Build history of the part. All positions in model axes, mm. A direction names the side the tool comes from. Coordinates: 2 decimals unless noted, no trailing zeros. Write item = value, one per line. Start each with the question number.
Q1. 3-axis set-ups, long thin cutter, end or side, ignore diameter. For faces 4 (the face through (-9.563, -21.028, 0.601)), 5 (the face through (9.854, -21.197, 6.399)), 6 (the face through (13.43, 19.13, 6.4)), 7 (the face through (-13.43, 18.8, 0.6)), 8 (the face through (9.78, -21.81, 3.48)): which of +Z, -Z, +X, -X, +Y, -Y reach the whole face in a straight line?
Q2. Band-saw the part on A-A on z = 6. State how many separate pieces and enclosed holes the cut face has, plus the area to 3 significant figures.
Q3. Drill centre lines: probe 1 along Y at (x, z) = (-0.5, 5.25); probe 2 along Y at (x, z) = (-10, 2.25); probe 3 along Y at (x, z) = (3, 5.25). Where is each one in solid material? Low to high.
Q4. Pin check, flat tips, straight feed: P1, Ø0.7, axis at x = 14.5, z = 3.5, coming from the +Y side; P2, Ø1.1, axis at y = -6.5, z = 3.5, coming from the -X side; P3, Ø1.1, axis at y = 15, z = 3, coming from the -X side; P4, Ø13, axis at x = -26.85, y = -15.5, coming from the +Z side. Stop position of each tip, or through.
Q5. Pull direction X, two halves, no side cores. Call faces 1 (the face through (9.854, -21.197, 0.601)), 2 (the face through (-13.43, 18.8, 6.4)), 3 (the face through (14, 19, 3)): released by +X, released by -X, zero draft, split by the parting line, or undercut.
```python
from build123d import *

# Parameters (mm, degrees)
F0_W     = 1.3256371551
F0_H     = 1.3256371551
F1_DEPTH = 7
F2_R     = 2


with BuildPart() as f1:
    # F0 (on Top) → F1 (new body)
    with BuildSketch(Plane.XY):
        with BuildLine():
            Line((0, 20.1), (0, 17))
            ThreePointArc((0, 17), (9.8994949366, 21.1005050634), (14, 31))
            ThreePointArc((14, 31), (9.8994949366, 40.8994949366), (0, 45))
            Line((0, 45), (0, 41.9))
            ThreePointArc((0, 41.9), (7.7074639149, 38.7074639149), (10.9, 31))
            ThreePointArc((10.9, 31), (7.7074639149, 23.2925360851), (0, 20.1))
        make_face()
        with BuildLine():
            ThreePointArc((-14, 31), (-9.8994949366, 21.1005050634), (0, 17))
            Line((0, 17), (0, 20.1))
            ThreePointArc((0, 20.1), (-10.9, 31), (0, 41.9))
            Line((0, 41.9), (0, 45))
            ThreePointArc((0, 45), (-9.8994949366, 40.8994949366), (-14, 31))
        make_face()
        with BuildLine():
            Line((0, 11), (0, 14.1517119482))
            Line((0, 14.1517119482), (0, 15.4773491033))
            Line((0, 15.4773491033), (0, 17))
            ThreePointArc((0, 17), (-9.8994949366, 21.1005050634), (-14, 31))
            Line((-14, 31), (-14, 8.0829037687))
            Line((-14, 8.0829037687), (-14, 0))
            Line((-14, 0), (-11, 0))
            ThreePointArc((-11, 0), (-7.7781745931, 7.7781745931), (0, 11))
        make_face()
        with BuildLine():
            Line((1.3256371551, 14.1517119482), (0, 14.1517119482))
            Line((0, 14.1517119482), (0, 11))
            ThreePointArc((0, 11), (7.7781745931, 7.7781745931), (11, 0))
            Line((11, 0), (14, 0))
            Line((14, 0), (14, 8.0829037687))
            Line((14, 8.0829037687), (14, 31))
            ThreePointArc((14, 31), (9.8994949366, 21.1005050634), (0, 17))
            Line((0, 17), (0, 15.4773491033))
            Line((0, 15.4773491033), (1.3256371551, 15.4773491033))
            Line((1.3256371551, 15.4773491033), (1.3256371551, 14.1517119482))
        make_face()
        with BuildLine():
            Line((14, 0), (11, 0))
            ThreePointArc((11, 0), (10.6251840892, -2.8470094961), (9.5262794416, -5.5))
            Line((9.5262794416, -5.5), (12.8533530208, -7.4208868265))
            Line((12.8533530208, -7.4208868265), (14.7224318643, -8.5))
            ThreePointArc((14.7224318643, -8.5), (23.2233210418, -1.9770383902), (33.8467877969, -3.3756445084))
            Line((33.8467877969, -3.3756445084), (14, 8.0829037687))
            Line((14, 8.0829037687), (14, 0))
        make_face()
        with Locations((13.5161715983, -6.758068249)):
            Rectangle(F0_W, F0_H, mode=Mode.SUBTRACT)
        with Locations((14.4693469893, -3.9606061499)):
            Rectangle(F0_W, F0_H, mode=Mode.SUBTRACT)
        with BuildLine():
            Line((12.8533530208, -7.4208868265), (9.5262794416, -5.5))
            ThreePointArc((9.5262794416, -5.5), (0, -11), (-9.5262794416, -5.5))
            Line((-9.5262794416, -5.5), (-14, -8.0829037687))
            Line((-14, -8.0829037687), (0, -16.1658075373))
            Line((0, -16.1658075373), (19.8467879874, -27.6243559244))
            ThreePointArc((19.8467879874, -27.6243559244), (13.3238260195, -19.1234668936), (14.7224318643, -8.5))
            Line((14.7224318643, -8.5), (12.8533530208, -7.4208868265))
        make_face()
        with BuildLine():
            ThreePointArc((-9.5262794416, -5.5), (-10.6251840892, -2.8470094961), (-11, 0))
            Line((-11, 0), (-14, 0))
            Line((-14, 0), (-14, 8.0829037687))
            Line((-14, 8.0829037687), (-33.8467875831, -3.375644385))
            ThreePointArc((-33.8467875831, -3.375644385), (-23.2233209225, -1.9770384221), (-14.7224318643, -8.5))
            Line((-14.7224318643, -8.5), (-14, -8.0829037687))
            Line((-14, -8.0829037687), (-9.5262794416, -5.5))
        make_face()
        with BuildLine():
            Line((0, -16.1658075373), (-14, -8.0829037687))
            Line((-14, -8.0829037687), (-14.7224318643, -8.5))
            ThreePointArc((-14.7224318643, -8.5), (-13.3238259493, -11.8765333686), (-12.8467875173, -15.5))
            ThreePointArc((-12.8467875173, -15.5), (-14.7224317836, -22.4999998602), (-19.8467872378, -27.6243554916))
            Line((-19.8467872378, -27.6243554916), (0, -16.1658075373))
        make_face()
        with Locations((-10.3011047203, -16.1628185775)):
            Rectangle(F0_W, F0_H, mode=Mode.SUBTRACT)
        with Locations((-8.161916424, -14.8371814225)):
            Rectangle(F0_W, F0_H, mode=Mode.SUBTRACT)
        with Locations((-10.4326661411, -13.3934514332)):
            Rectangle(F0_W, F0_H, mode=Mode.SUBTRACT)
        with BuildLine():
            ThreePointArc((-12.8467875173, -15.5), (-13.3238259493, -11.8765333686), (-14.7224318643, -8.5))
            Line((-14.7224318643, -8.5), (-17.5803156968, -10.15))
            ThreePointArc((-17.5803156968, -10.15), (-16.511381176, -12.7306362174), (-16.1467875173, -15.5))
            ThreePointArc((-16.1467875173, -15.5), (-24.0774237347, -25.8354063413), (-36.1132593378, -20.85))
            Line((-36.1132593378, -20.85), (-38.9711431703, -22.5))
            ThreePointArc((-38.9711431703, -22.5), (-30.4702539929, -29.0229616098), (-19.8467872378, -27.6243554916))
            ThreePointArc((-19.8467872378, -27.6243554916), (-14.7224317836, -22.4999998602), (-12.8467875173, -15.5))
        make_face()
        with BuildLine():
            ThreePointArc((-14.7224318643, -8.5), (-23.2233209225, -1.9770384221), (-33.8467875831, -3.375644385))
            ThreePointArc((-33.8467875831, -3.375644385), (-40.3697490952, -11.8765334052), (-38.9711431703, -22.5))
            Line((-38.9711431703, -22.5), (-36.1132593378, -20.85))
            ThreePointArc((-36.1132593378, -20.85), (-32.1967875173, -6.2335281795), (-17.5803156968, -10.15))
            Line((-17.5803156968, -10.15), (-14.7224318643, -8.5))
        make_face()
        with BuildLine():
            ThreePointArc((40.8467875173, -15.5), (38.971143251, -8.5000001398), (33.8467877969, -3.3756445084))
            ThreePointArc((33.8467877969, -3.3756445084), (23.2233210418, -1.9770383902), (14.7224318643, -8.5))
            Line((14.7224318643, -8.5), (17.4937131564, -10.1))
            ThreePointArc((17.4937131564, -10.1), (29.6420332044, -5.0680010761), (37.6467875173, -15.5))
            ThreePointArc((37.6467875173, -15.5), (37.2787864412, -18.2952456871), (36.1998618782, -20.9))
            Line((36.1998618782, -20.9), (38.9711431703, -22.5))
            ThreePointArc((38.9711431703, -22.5), (40.3697490854, -19.1234666314), (40.8467875173, -15.5))
        make_face()
        with BuildLine():
            Line((17.4937131564, -10.1), (14.7224318643, -8.5))
            ThreePointArc((14.7224318643, -8.5), (13.3238260195, -19.1234668936), (19.8467879874, -27.6243559244))
            ThreePointArc((19.8467879874, -27.6243559244), (30.4702544109, -29.0229614978), (38.9711431703, -22.5))
            Line((38.9711431703, -22.5), (36.1998618782, -20.9))
            ThreePointArc((36.1998618782, -20.9), (21.4467875173, -24.8530743609), (17.4937131564, -10.1))
        make_face()
    extrude(amount=F1_DEPTH)

    # F2
    f2_edges = [f1.edges().sort_by_distance(p)[0] for p in [
        (-14, 19.541452, 7),
        (0, 45, 7),
        (-23.923394, 2.35363, 7),
        (-38.971143, -22.5, 7),
        (-9.923394, -21.895082, 7),
        (9.923394, -21.895082, 7),
        (38.971143, -22.5, 7),
        (23.923394, 2.35363, 7),
        (14, 19.541452, 7),
        (-9.923394, -21.895082, 0),
        (-38.971143, -22.5, 0),
        (9.923394, -21.895082, 0),
        (38.971143, -22.5, 0),
        (23.923394, 2.35363, 0),
        (14, 19.541452, 0),
        (0, 45, 0),
    ]]
    fillet(f2_edges, radius=F2_R)


solid = f1.part
```
Recorded:
q1.face_4 = -Z, -Y
q1.face_5 = +Z, -Y
q1.face_6 = +Z, +X, +Y
q1.face_7 = -Z, -X, +Y
q1.face_8 = +Z, -Z, -Y
q2.separate_pieces = 1
q2.enclosed_holes = 10
q2.area = 1,630 mm2
q3.probe_1 = -16.44 to -10.99, 10.99 to 20.11, 41.89 to 44.98
q3.probe_2 = -21.94 to -16.83, -15.5 to -14.06, -12.73 to -4.58, 4.58 to 26.66, 35.34 to 40.8
q3.probe_3 = -17.88 to -10.58, 10.58 to 20.52, 41.48 to 44.66
q4.P1 = 8
q4.P2 = -38.01
q4.P3 = -14
q4.P4 = through
q5.face_1 = undercut
q5.face_2 = released by -X
q5.face_3 = released by +X
